from build123d import *

# Parameters (mm, degrees)
SKETCH_1_W             = 22.5
SKETCH_1_H             = 17
EXTRUDE_1_DEPTH        = 6.5
SKETCH_2_W             = 3.3
SKETCH_2_H             = 7
CUT_EXTRUDE_1_DEPTH    = 23.5
HOLE_WIZARD_M2_1_D     = 1.6
HOLE_WIZARD_M2_1_DEPTH = 10.1
HOLE_WIZARD_M2_1_TIP   = 0.480688495


with BuildPart() as part:
    # 草图1 → 凸台-拉伸1 (new body)
    with BuildSketch(Plane.XY):
        with Locations((11.25, 8.5)):
            Rectangle(SKETCH_1_W, SKETCH_1_H)
    extrude(amount=EXTRUDE_1_DEPTH)

    # 草图2 → 切除-拉伸1 (cut, through all)
    with BuildSketch(Plane.ZY):
        with Locations((4.85, 8.5)):
            Rectangle(SKETCH_2_W, SKETCH_2_H)
    extrude(amount=-CUT_EXTRUDE_1_DEPTH, mode=Mode.SUBTRACT)

    # M2 螺纹孔1
    with Locations(Plane(origin=(0, 0, 0), x_dir=(-1, 0, 0), z_dir=(0, 0, -1))):
        with Locations((-15.25, 2.5), (-7.25, 2.5), (-15.25, 14.5), (-7.25, 14.5)):
            Hole(HOLE_WIZARD_M2_1_D / 2, depth=HOLE_WIZARD_M2_1_DEPTH)
            with Locations((0, 0, -(HOLE_WIZARD_M2_1_DEPTH + HOLE_WIZARD_M2_1_TIP / 2))):  # 118° drill point
                Cone(0, HOLE_WIZARD_M2_1_D / 2, HOLE_WIZARD_M2_1_TIP, mode=Mode.SUBTRACT)


solid = part.part
Here's how the part is built. I have some questions about the finished solid (model axes, mm). A direction names the side the tool comes from. Give positions to 0.01 mm unless a question says otherwise; leave off trailing zeros. Order: outer loops, then holes, each group sorted by start corner. A loop starts at its lowest first (then second) coordinate and runs counter-clockwise, first axis right, second up. Notation, with made-up numbers: (-35.5, 75.5) -> (23.5, 75.5) arc R7 ccw to (23.5, 81.5) -> close; hole circle Ø6 at (-29.5, 59.25). An arc over 180 degrees is marked (long way). Use a Markdown table: item, result. Add a question column.
Item 1: Imagine slicing it at A-A on z = 4. Please give me the cut outline in (x, y).
Item 2: For faces 1 (the face through (11, 9, 0)), 2 (the face through (11, 8, 3.2)), which set-ups out of +Z, -Z, +X, -X, +Y, -Y let a thin tool reach every point of the face, with its end or its side?
Item 3: Imagine slicing it at D-D on y = 9.25. Please give me the cut outline in (x, z), plus the area to 3 significant figures.
Item 4: I need wall thicknesses on line 1 (Y direction, x = 15.25, z = 3); line 2 (Y direction, x = 17.75, z = 5.25); line 3 (Z direction, x = 17.5, y = 5.5). Which ranges of each line are inside material? Lowest first, please.
Item 5: Imagine slicing it at C-C on x = 15.25. Please give me the cut outline in (y, z), plus the area to 3 significant figures.
Item 6: Will these pins go through, and if not, where does the flat tip stop? pin 1 (1.5 mm diameter, centred on y = 13.5, z = 5.5, fed in from -X); pin 2 (1 mm diameter, centred on x = 7.25, y = 2.5, fed in from +Z); pin 3 (2 mm diameter, centred on x = 6, y = 7.5, fed in from +Z).
Item 7: Imagine slicing it at B-B on y = 14.5. Please give me the cut outline in (x, z), plus the area to 3 significant figures.
Data:
| question | item | result |
|---|---|---|
| 1 | outline | (0, 0) -> (22.5, 0) -> (22.5, 5) -> (0, 5) -> close; (0, 12) -> (22.5, 12) -> (22.5, 17) -> (0, 17) -> close; hole circle Ø1.6 at (7.25, 2.5); hole circle Ø1.6 at (7.25, 14.5); hole circle Ø1.6 at (15.25, 2.5); hole circle Ø1.6 at (15.25, 14.5) |
| 2 | face 1 | -Z, +X, -X, +Y, -Y |
| 2 | face 2 | +Z, +X, -X |
| 3 | outline | (0, 0) -> (22.5, 0) -> (22.5, 3.2) -> (0, 3.2) -> close |
| 3 | area | 72.0 mm² |
| 4 | line 1 | y = 0 to 1.7, 3.3 to 13.7, 15.3 to 17 |
| 4 | line 2 | y = 0 to 5, 12 to 17 |
| 4 | line 3 | z = 0 to 3.2 |
| 5 | outline | (0, 0) -> (1.7, 0) -> (1.7, 6.5) -> (0, 6.5) -> close; (3.3, 0) -> (13.7, 0) -> (13.7, 6.5) -> (12, 6.5) -> (12, 3.2) -> (5, 3.2) -> (5, 6.5) -> (3.3, 6.5) -> close; (15.3, 0) -> (17, 0) -> (17, 6.5) -> (15.3, 6.5) -> close |
| 5 | area | 66.6 mm² |
| 6 | pin 1 | stops at x = 0 |
| 6 | pin 2 | passes through |
| 6 | pin 3 | stops at z = 3.2 |
| 7 | outline | (0, 0) -> (6.45, 0) -> (6.45, 6.5) -> (0, 6.5) -> close; (8.05, 0) -> (14.45, 0) -> (14.45, 6.5) -> (8.05, 6.5) -> close; (16.05, 0) -> (22.5, 0) -> (22.5, 6.5) -> (16.05, 6.5) -> close |
| 7 | area | 125 mm² |
